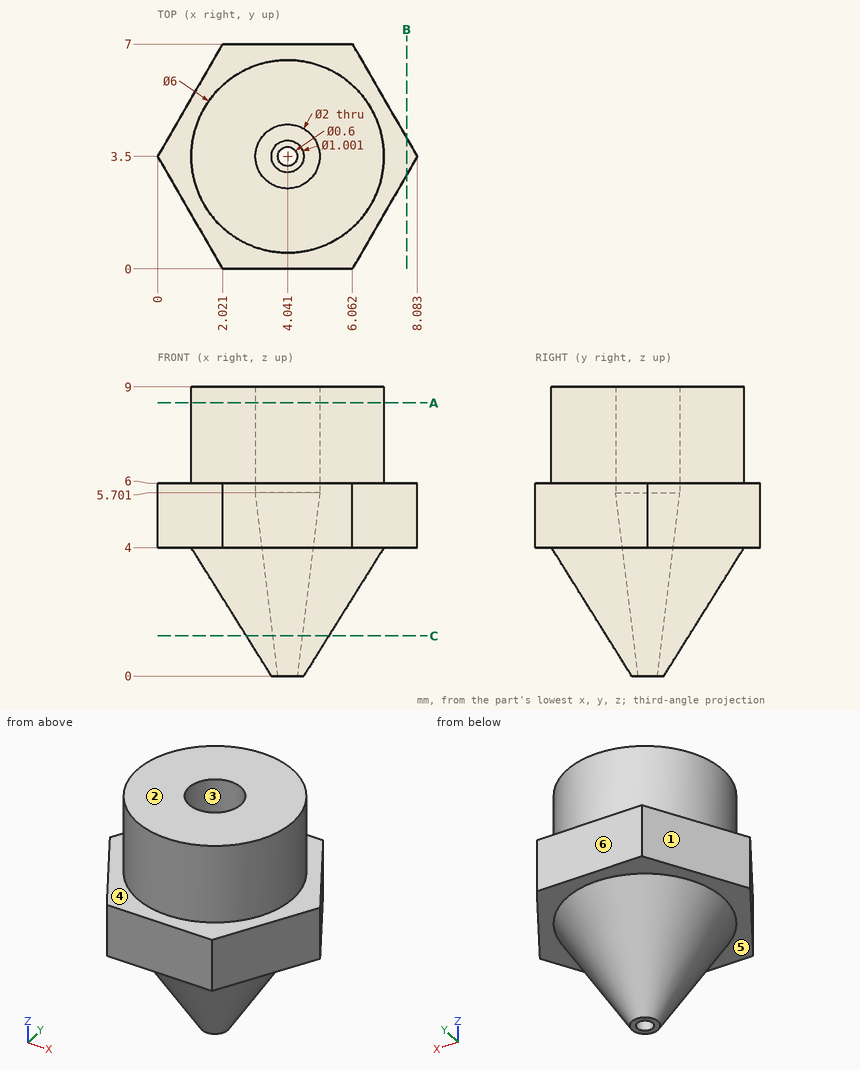
The drawing under review shows one solid part. Ordinate dimensions are in mm from its lowest x, y, z. A direction names the side the tool comes from. Coordinates: 2 decimals unless noted, no trailing zeros. Loops run counter-clockwise (first coordinate to the right, second up) from the corner with the lowest first, then second, coordinate; pieces in that order, holes last. Notation, with made-up numbers: M 24.5,70.25 L 53.5,70.25 A22 cw 53.5,93.25 Z; hole C -13.75,-26.75 d3. An arc over 180 degrees is marked long. Use one line per item in the form item = value.
(1) Draft analysis for pull direction Y (two halves, no side actions). For the marked faces 1, 2 and 3, state which applies: pulls with the +Y half, pulls with the -Y half, needs draft (parallel to the pull), parting line crosses it, or undercut.
Return value:
face_1 = pulls with the +Y half
face_2 = needs draft
face_3 = undercut
(2) Consider section B-B (x = 7.75). Write out the cut boundary in (y, z).
Return value:
outline = M 2.92,4 L 4.08,4 L 4.08,6 L 2.92,6 Z
(3) For line 1 along Z through (x, y) = (1.5, 5.5); line 2 along Y through (x, z) = (4.25, 7.5); line 3 along X through (y, z) = (3, 7.25) (1 decimal), list the stretches that pass through material, from the lowest coordinate up. Write a range as from..to.
Return value:
line_1 = 4..6
line_2 = 0.51..2.52, 4.48..6.49
line_3 = 1.1..3.2, 4.9..7
(4) For the marked faces 4, 5 and 6, list the 3-axis set-ups (+Z, -Z, +X, -X, +Y, -Y) from which the entire face can be reached by the end or side of a thin tool; tool diameter is ignored.
Return value:
face_4 = +Z
face_5 = -Z
face_6 = +Z, -Z, +X, -X, +Y
(5) Consider section A-A (z = 8.5). Write out the cut boundary in (x, y).
Return value:
outline = C 4.04,3.5 d6; hole C 4.04,3.5 d2
(6) Consider section C-C (z = 1.25). Write out the cut boundary in (x, y) (1 decimal).
Return value:
outline = C 4,3.5 d2.6; hole C 4,3.5 d0.9
